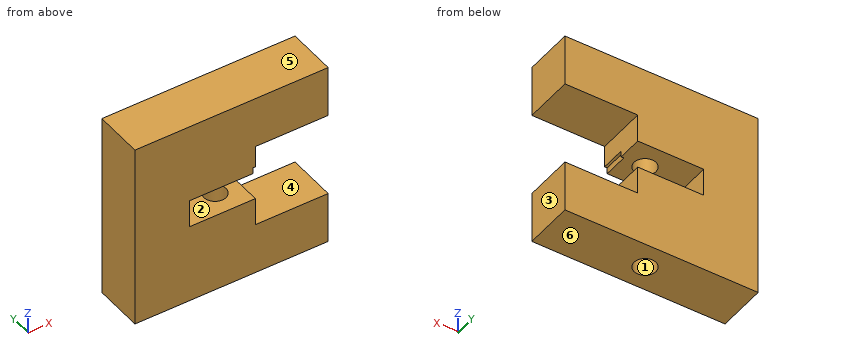
from build123d import *

# Parameters (mm, degrees)
F0_W     = 873.76
F0_H     = 848.36
F1_DEPTH = 223.52
F3_DEPTH = 254
F5_D     = 75
F5_DEPTH = 675.64
F5_TIP   = 22.5322732135
F7_W     = 22.5396603346
F7_H     = 45.0793132186
F8_DEPTH = 111.76


with BuildPart() as f1:
    # F0 (on Front) → F1 (new body)
    with BuildSketch(Plane.XZ):
        Rectangle(F0_W, F0_H)
    extrude(amount=F1_DEPTH)

    # F2 (on face) → F3 (cut)
    with BuildSketch(Plane.XZ.offset(223.52)):
        Polygon((107.696, 85.352614522), (107.696, 63.5), (-190.5, 63.5), (-190.5, 48.8914474845), (-190.5, 0), (-190.5, -48.8914474845), (-190.5, -63.5), (107.696, -63.5), (107.696, -85.352614522), (107.696, -181.2319755554), (107.696, -190.5), (716.4556980133, -190.5), (716.4556980133, 190.5), (430.53, 190.5), (107.696, 190.5), (107.696, 181.2319755554), align=None)
    extrude(amount=-F3_DEPTH, mode=Mode.SUBTRACT)

    # F5
    with Locations(Plane(origin=(0, 0, -424.18), x_dir=(1, 0, 0), z_dir=(0, 0, -1))):
        with Locations((0, 111.76)):
            Hole(F5_D / 2, depth=F5_DEPTH)
            with Locations((0, 0, -(F5_DEPTH + F5_TIP / 2))):  # 118° drill point
                Cone(0, F5_D / 2, F5_TIP, mode=Mode.SUBTRACT)

    # F7 (on face) → F8 (cut)
    with BuildSketch(Plane.XZ.offset(223.52)):
        with Locations((107.1918830276, 69.2144595087)):
            Rectangle(F7_W, F7_H)
    extrude(amount=-F8_DEPTH, mode=Mode.SUBTRACT)

    # F9 (on offset) → F10 (revolve, cut)
    with BuildSketch(Plane.XZ.offset(111.76)):
        Polygon((8.588981392, -428.1635656953), (49.5, -428.1635656953), (49.5, 249.0316255649), (37.7547182143, 251.635491848), (18.8773591071, 251.635491848), align=None)
    revolve(axis=Axis((0, -111.76, 257.2192468215), (0, 0, 1)), mode=Mode.SUBTRACT)


solid = f1.part
The listing builds one solid part. Answer for the finished solid, in the listing's coordinates (mm). Face numbers are marked on the shaded views. A direction names the side the tool comes from. Round coordinates to 2 decimals unless told otherwise and drop trailing zeros. Loops run counter-clockwise (first coordinate to the right, second up) from the corner with the lowest first, then second, coordinate; pieces in that order, holes last. Notation, with made-up numbers: M 54,20.25 L 76,20.25 A29 cw 76,44.25 Z; hole C 88.25,51 d8. An arc over 180 degrees is marked long. Return JSON: item names as keys, results as strings.
Q1. Find section B-B, the plane y = -49.5. Determine the outline of the cut face in (x, z).
Results list:
{"outline": "M -436.88,-424.18 L 436.88,-424.18 L 436.88,-190.5 L 107.7,-190.5 L 107.7,-63.5 L -190.5,-63.5 L -190.5,63.5 L 107.7,63.5 L 107.7,190.5 L 436.88,190.5 L 436.88,424.18 L -436.88,424.18 Z"}
Q2. Find section A-A, the plane x = 341.5. Determine the outline of the cut face in (y, z), plus the area to 3 significant figures.
Results list:
{"outline": "M -223.52,-424.18 L 0,-424.18 L 0,-190.5 L -223.52,-190.5 Z; M -223.52,190.5 L 0,190.5 L 0,424.18 L -223.52,424.18 Z", "area": "104,000 mm2"}
Q3. This flat-tipped pin is pushed along its axis until it touches: pin 1 Ø3.5 at (x, z) = (104.5, 76) entering from -Y. Where does it stop, or does it pass through?
Results list:
{"pin 1": "stops at y = -111.76"}
Q4. Which of the six approach directions +Z, -Z, +X, -X, +Y, -Y give full straight-line access (tool end or side, diameter ignored) to the marked faces 1, 2 and 3?
Results list:
{"face 1": "-Z", "face 2": "+X, +Y, -Y", "face 3": "+Z, -Z, +X, +Y, -Y"}
Q5. Find section C-C, the plane z = -147.5. Determine the outline of the cut face in (x, y), plus the area to 3 significant figures.
Results list:
{"outline": "M -436.88,-223.52 L 107.7,-223.52 L 107.7,0 L -436.88,0 Z; hole C 0,-111.76 d99", "area": "114,000 mm2"}
Q6. Find the intervals of material crossed by line 1 along Z through (x, y) = (-57, -60); line 2 along Y through (x, z) = (0, 151); line 3 along X through (y, z) = (-111, 105), in increasing order. Write a range as from..to.
Results list:
{"line 1": "z = -424.18..-63.5, 63.5..424.18", "line 2": "y = -223.52..-161.26, -62.26..0", "line 3": "x = -436.88..-49.49, 49.49..107.7"}
Q7. The mould has two halves that part along Z. Classify the marked faces 4, 5 and 6: released by +Z, released by -Z, zero draft, split by the parting line, or undercut.
Results list:
{"face 4": "undercut", "face 5": "released by +Z", "face 6": "released by -Z"}
